Autodesk Inventor part; units mm, degrees
ref_plane "YZ Plane" through (0, 0, 0) normal (1, 0, 0) x (0, 1, 0)
ref_plane "XZ Plane" through (0, 0, 0) normal (0, 1, 0) x (-1, 0, 0)
ref_plane "XY Plane" through (0, 0, 0) normal (0, 0, 1) x (1, 0, 0)
sketch "Sketch1" plane through (0, 0, 0) normal (0, 1, 0) x (-1, 0, 0)
  circle A0 centre (0, 0) radius 18.85
  circle A1 centre (0, 0) radius 2.75
  dimension "d0" = 37.7
  dimension "d1" = 5.5
extrude "Extrusion1" add sketch "Sketch1" along normal blind 11
sketch "Sketch2" plane through (0, 11, 0) normal (0, 1, 0) x (1, 0, 0)
  circle A0 centre (0, 0) radius 20
  circle A1 centre (0, 0) radius 18.85
  dimension "d4" = 40
extrude "Extrusion2" add sketch "Sketch2" against normal blind 2
sketch "Sketch3" plane through (0, 0, 0) normal (0, -1, 0) x (1, 0, 0)
  circle A0 centre (0, 0) radius 20
  circle A1 centre (0, 0) radius 18.85
  dimension "d7" = 40
  dimension "d8" = 37.7
extrude "Extrusion3" add sketch "Sketch3" against normal blind 2
sketch "Sketch4" plane through (0, 0, 0) normal (0, -1, 0) x (1, 0, 0)
  circle A0 centre (0, 0) radius 10
  circle A1 centre (0, 0) radius 2.75
  dimension "d11" = 20
  dimension "d12" = 5.5
extrude "Extrusion4" add sketch "Sketch4" along normal blind 7
Model file for the job. Use its own axes, mm. A direction names the side the tool comes from. Round coordinates to 2 decimals unless told otherwise and drop trailing zeros. Order: outer loops, then holes, each group sorted by start corner. A loop starts at its lowest first (then second) coordinate and runs counter-clockwise, first axis right, second up. Notation, with made-up numbers: (42.5, 86.5) -> (83.5, 86.5) arc R25 cw to (83.5, 116.5) -> close; hole circle Ø2 at (-9, -28.5). An arc over 180 degrees is marked (long way). Use one line per item in the form item = value.
Item 1: Cut at C-C, the plane y = -4.75. Write the cut outline in (x, z).
Returned:
outline = circle Ø20 at (0, 0); hole circle Ø5.5 at (0, 0)
Item 2: Cut at D-D, the plane x = 12. Write the cut outline in (y, z).
Returned:
outline = (0, -16) -> (2, -16) -> (2, -14.54) -> (9, -14.54) -> (9, -16) -> (11, -16) -> (11, 16) -> (9, 16) -> (9, 14.54) -> (2, 14.54) -> (2, 16) -> (0, 16) -> close
Item 3: Drill centre lines: line 1 (X direction, y = 7.5, z = 0); line 2 (X direction, y = 10, z = 0). Where is each one in solid material? Low to high.
Returned:
line_1 = -18.85 to -2.75, 2.75 to 18.85
line_2 = -20 to -2.75, 2.75 to 20
Item 4: Cut at A-A, the plane x = 0. Write the cut outline in (y, z).
Returned:
outline = (-7, -10) -> (0, -10) -> (0, -20) -> (2, -20) -> (2, -18.85) -> (9, -18.85) -> (9, -20) -> (11, -20) -> (11, -2.75) -> (-7, -2.75) -> close; (-7, 2.75) -> (11, 2.75) -> (11, 20) -> (9, 20) -> (9, 18.85) -> (2, 18.85) -> (2, 20) -> (0, 20) -> (0, 10) -> (-7, 10) -> close
Item 5: Tool access for faces 5 (the face through (-4.336, 10.014, 19.524)), 6 (the face through (-15, 9, -12)), 7 (the face through (-5, 0, 9)): list every direction of +Z, -Z, +X, -X, +Y, -Y with a clear straight run to the whole face (end or side of a thin tool).
Returned:
face_5 = +Y, -Y
face_6 = none
face_7 = -Y
Item 6: Cut at B-B, the plane z = 0. Write the cut outline in (x, y).
Returned:
outline = (-20, 0) -> (-10, 0) -> (-10, -7) -> (-2.75, -7) -> (-2.75, 11) -> (-20, 11) -> (-20, 9) -> (-18.85, 9) -> (-18.85, 2) -> (-20, 2) -> close; (2.75, -7) -> (10, -7) -> (10, 0) -> (20, 0) -> (20, 2) -> (18.85, 2) -> (18.85, 9) -> (20, 9) -> (20, 11) -> (2.75, 11) -> close
Item 7: Pull direction Y, two halves, no side cores. Call faces 1 (the face through (-4.336, 0.986, -19.524)), 2 (the face through (2.1, -7, -2.1)), 3 (the face through (-4, 11, 0)), 4 (the face through (4.1, 5.5, 18.4)): released by +Y, released by -Y, zero draft, split by the parting line, or undercut.
Returned:
face_1 = zero draft
face_2 = released by -Y
face_3 = released by +Y
face_4 = undercut
Item 8: Flat gauge pins, fed straight in: pin 1 Ø8 at (y, z) = (5.5, -11) entering from -X; pin 2 Ø6 at (x, y) = (-10, 1.5) entering from -Z (3 decimals); pin 3 Ø2 at (x, y) = (7, -5) entering from +Z. Where does each tip first touch, or does it go through?
Returned:
pin_1 = -17.83
pin_2 = -18.735
pin_3 = 8
